```python
from build123d import *

# Parameters (mm, degrees)
BOSS_EXTRUDE1_DEPTH = 230
SKETCH2_R           = 4
CUT_EXTRUDE1_DEPTH  = 241.62418831


with BuildPart() as part:
    # Sketch1 → Boss-Extrude1 (new body)
    with BuildSketch(Plane.XY):
        Polygon((0, 0), (0, 50), (-5, 50), (-5, 0), (-5, -5), (50, -5), (50, 0), align=None)
    extrude(amount=BOSS_EXTRUDE1_DEPTH)

    # Sketch2 → Cut-Extrude1 (cut, through all)
    with BuildSketch(Plane(origin=(0, 0, 0), x_dir=(0, 0, -1), z_dir=(1, 0, 0))):
        with Locations((-115, 25)):
            Circle(SKETCH2_R)
        with Locations((-25, 25)):
            Circle(SKETCH2_R)
        with Locations((-205, 25)):
            Circle(SKETCH2_R)
    extrude(amount=-CUT_EXTRUDE1_DEPTH, mode=Mode.SUBTRACT)


solid = part.part
```
The model under review builds one solid part; all positions refer to its coordinate system, in mm. Give positions to 0.01 mm unless a question says otherwise; leave off trailing zeros. Loops run counter-clockwise (first coordinate to the right, second up) from the corner with the lowest first, then second, coordinate; pieces in that order, holes last. Notation, with made-up numbers: (-32, 37.25) - (13, 37.25) arc R17 cw to (13, 41.25) - close; hole circle Ø8 at (-16.5, 47.5). An arc over 180 degrees is marked (long way). Answer as a JSON object with one key per item and string values.
Q1. Add section D-D on x = 23.5. State the section outline as (y, z) points.
Worked out:
{"outline": "(-5, 0) - (0, 0) - (0, 230) - (-5, 230) - close"}
Q2. Mouldability with a two-part tool opening along Y and no side actions: class faces 1 (the cylindrical face through (-2.465, 26.201, 111.185)), 2 (the flat face through (25, 0, 113)), 3 (the flat face through (22, -5, 113)), 4 (the flat face through (0, 19, 113)) as +Y half, -Y half, draft (parallel to the pull), parting line (faces both ways), or undercut.
Worked out:
{"face 1": "undercut", "face 2": "+Y half", "face 3": "-Y half", "face 4": "draft"}
Q3. Add section A-A on z = 25. State the section outline as (x, y) points.
Worked out:
{"outline": "(-5, -5) - (50, -5) - (50, 0) - (0, 0) - (0, 21) - (-5, 21) - close; (-5, 29) - (0, 29) - (0, 50) - (-5, 50) - close"}
Q4. Add section C-C on z = 51. State the section outline as (x, y) points, plus the area to 3 significant figures.
Worked out:
{"outline": "(-5, -5) - (50, -5) - (50, 0) - (0, 0) - (0, 50) - (-5, 50) - close", "area": "525 mm^2"}
Q5. Add section B-B on y = 23. State the section outline as (x, z) points, plus the area to 3 significant figures.
Worked out:
{"outline": "(-5, 0) - (0, 0) - (0, 21.54) - (-5, 21.54) - close; (-5, 28.46) - (0, 28.46) - (0, 111.54) - (-5, 111.54) - close; (-5, 118.46) - (0, 118.46) - (0, 201.54) - (-5, 201.54) - close; (-5, 208.46) - (0, 208.46) - (0, 230) - (-5, 230) - close", "area": "1,050 mm^2"}
Q6. Insertion check: pin 1 (9 mm diameter, centred on y = 25, z = 25, fed in from +X); pin 2 (6 mm diameter, centred on x = 35.5, z = 50.5, fed in from +Y). Each pin has a flat end and moves straight along its axis. Give the tip position at first contact, or say it passes through.
Worked out:
{"pin 1": "stops at x = 0", "pin 2": "stops at y = 0"}
Q7. To check wall thickness, follow line 1 along Y through (x, z) = (-2, 25); line 2 along Y through (x, z) = (11, 117.5). State the ranges of each line that lie inside material, in increasing order.
Worked out:
{"line 1": "y = -5 to 21, 29 to 50", "line 2": "y = -5 to 0"}
